from build123d import *

# Parameters (mm, degrees)
SKETCH1_R               = 17.4625
BOSS_EXTRUDE1_DEPTH     = 5
BOSS_EXTRUDE2_START     = 127
SKETCH1_2_R             = 17.4625
BOSS_EXTRUDE2_DEPTH     = 5
BOSS_EXTRUDE3_DEPTH     = 122
SKETCH3_W               = 34.925
SKETCH3_H               = 82
CUT_EXTRUDE1_DEPTH      = 18.4625
CUT_EXTRUDE1_DEPTH_BACK = 18.4625


with BuildPart() as part:
    # Sketch1 → Boss-Extrude1 (new body)
    with BuildSketch(Plane(origin=(0, 0, 0), x_dir=(1, 0, 0), z_dir=(0, 1, 0))):
        Circle(SKETCH1_R)
    extrude(amount=BOSS_EXTRUDE1_DEPTH)



with BuildPart() as body_2:
    # Sketch1<2> → Boss-Extrude2 (new body)
    with BuildSketch(Plane(origin=(0, 0, 0), x_dir=(1, 0, 0), z_dir=(0, 1, 0)).offset(BOSS_EXTRUDE2_START)):
        Circle(SKETCH1_2_R)
    extrude(amount=BOSS_EXTRUDE2_DEPTH)


with BuildPart() as part_1:
    add(part.part)

    add(body_2.part)  # Boss-Extrude3 merges body 2
    # Sketch2 → Boss-Extrude3 (add)
    with BuildSketch(Plane(origin=(0, 5, 0), x_dir=(1, 0, 0), z_dir=(0, 1, 0))):
        with BuildLine():
            Line((-4.769696007, -1.5), (-1.5, -1.5))
            Line((-1.5, -1.5), (-1.5, -4.769696007))
            ThreePointArc((-1.5, -4.769696007), (0, -5), (1.5, -4.769696007))
            Line((1.5, -4.769696007), (1.5, -1.5))
            Line((1.5, -1.5), (4.769696007, -1.5))
            ThreePointArc((4.769696007, -1.5), (5, 0), (4.769696007, 1.5))
            Line((4.769696007, 1.5), (1.5, 1.5))
            Line((1.5, 1.5), (1.5, 4.769696007))
            ThreePointArc((1.5, 4.769696007), (0, 5), (-1.5, 4.769696007))
            Line((-1.5, 4.769696007), (-1.5, 1.5))
            Line((-1.5, 1.5), (-4.769696007, 1.5))
            ThreePointArc((-4.769696007, 1.5), (-5, 0), (-4.769696007, -1.5))
        make_face()
    extrude(amount=BOSS_EXTRUDE3_DEPTH)

    # Sketch3 → Cut-Extrude1 (cut, two sides)
    with BuildSketch(Plane.XY) as cut_extrude1_sk:
        with Locations((0, 91)):
            Rectangle(SKETCH3_W, SKETCH3_H)
    extrude(amount=CUT_EXTRUDE1_DEPTH, mode=Mode.SUBTRACT)
    extrude(cut_extrude1_sk.sketch, amount=-CUT_EXTRUDE1_DEPTH_BACK, mode=Mode.SUBTRACT)


solid = part_1.part
CAD build for the part. Positions are in the model's coordinates, mm. A direction names the side the tool comes from. Give positions to 0.01 mm unless a question says otherwise; leave off trailing zeros. Write each loop counter-clockwise with the first axis right and the second up, starting at its lowest first coordinate (ties: lowest second). Pieces come first, ordered by that corner, then holes. Notation, with made-up numbers: M 80.5,-25.5 L 134.5,-25.5 A24 cw 134.5,12.5 Z; hole C 66,39.5 d2. An arc over 180 degrees is marked long. Put each result on its own line as item: value. Start each with the question number.
(1) Band-saw the part on B-B, the plane x = 0. Write the cut outline in (y, z).
(2) Flat gauge pins, fed straight in: pin 1 Ø6 at (x, y) = (-9, 18) entering from -Z; pin 2 Ø2.5 at (x, y) = (3.5, 33) entering from -Z; pin 3 Ø3.5 at (x, y) = (2.5, 27) entering from +Z; pin 4 Ø12 at (x, z) = (-7.5, -12.5) entering from +Y. Where does each tip first touch, or does it go through?
(3) Which spindle directions (+Z, -Z, +X, -X, +Y, -Y) get a long thin tool onto all of the face, cutting with end or side? Do faces 1 (the face through (-5, 27, 0)), 2 (the face through (3, 27, -1.5)), 3 (the face through (-1.5, 27, -3)). Say none if no direction does.
(4) Band-saw the part on A-A, the plane y = 13. Write the cut outline in (x, z), and give its area (3 significant figures).
(5) Band-saw the part on D-D, the plane x = -15. Write the cut outline in (y, z).
(6) Probe L1, parallel to Y at x = 12, z = -4.5; L2, parallel to Z at x = 2, y = 35; L3, parallel to Z at x = -0.5, y = 28. List the from-to ranges inside material, lowest first.
(7) Band-saw the part on C-C, the plane z = 3. Write the cut outline in (x, y), and give its area (3 significant figures).
Response values:
1. outline: M 0,-17.46 L 5,-17.46 L 5,-5 L 50,-5 L 50,5 L 5,5 L 5,17.46 L 0,17.46 Z
2. pin 1: passes through
2. pin 2: stops at z = -1.5
2. pin 3: stops at z = 4.94
2. pin 4: stops at y = 5
3. face 1: -X, +Y
3. face 2: -Z, +X, +Y
3. face 3: -Z, -X, +Y
4. outline: M -4.77,-1.5 L -1.5,-1.5 L -1.5,-4.77 A5 ccw 1.5,-4.77 L 1.5,-1.5 L 4.77,-1.5 A5 ccw 4.77,1.5 L 1.5,1.5 L 1.5,4.77 A5 ccw -1.5,4.77 L -1.5,1.5 L -4.77,1.5 A5 ccw Z
4. area: 50.1 mm2
5. outline: M 0,-8.94 L 5,-8.94 L 5,8.94 L 0,8.94 Z
6. L1: y = 0 to 5
6. L2: z = -1.5 to 1.5
6. L3: z = -4.97 to 4.97
7. outline: M -17.2,0 L 17.2,0 L 17.2,5 L 1.5,5 L 1.5,50 L -1.5,50 L -1.5,5 L -17.2,5 Z
7. area: 307 mm2
